Answer from the drawing. Dimensions are ordinates in mm from the lowest x, y and z of the part. A direction names the side the tool comes from. Coordinates: 2 decimals unless noted, no trailing zeros. Order: outer loops, then holes, each group sorted by start corner. A loop starts at its lowest first (then second) coordinate and runs counter-clockwise, first axis right, second up. Notation, with made-up numbers: (80, 75) - (131, 75) arc R33 cw to (131, 103) - close; hole circle Ø9 at (-11.75, -1.5). An arc over 180 degrees is marked (long way). Use CSV: the item, a comma, the result in double quotes. Start each with the question number.
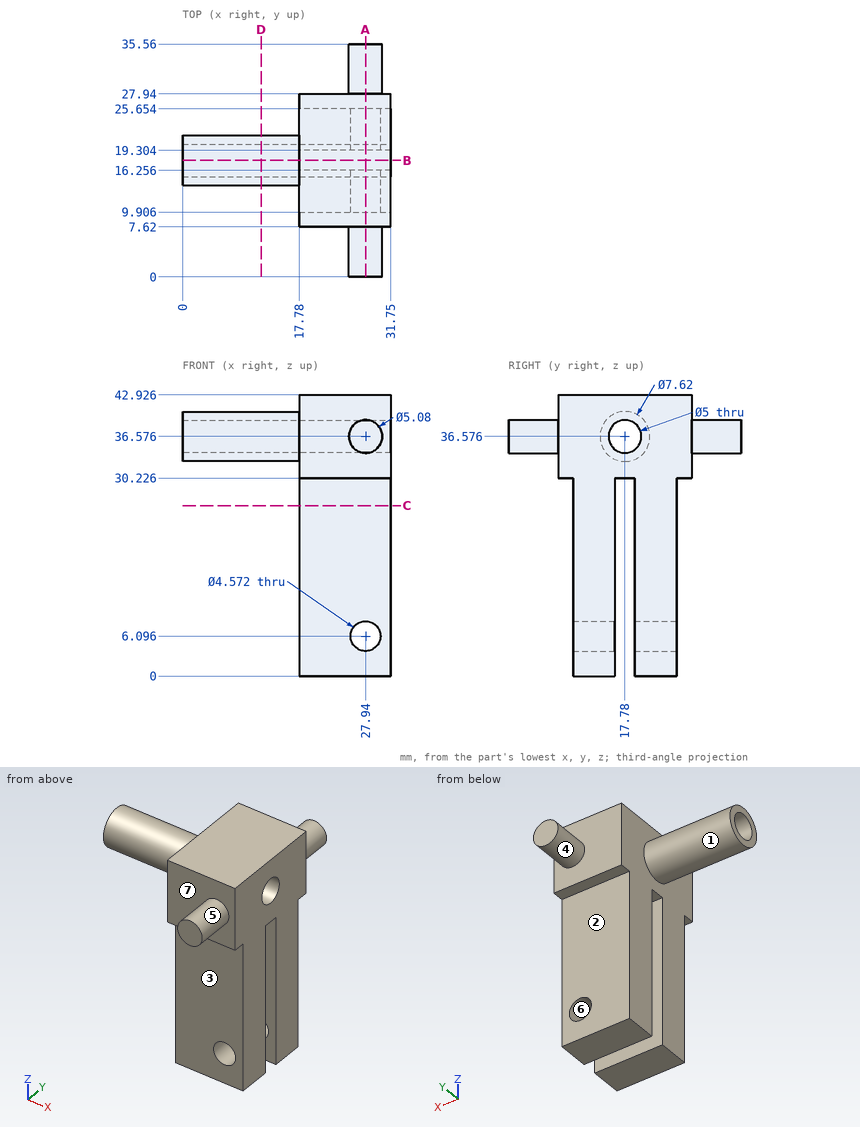
1) Straight lines are drawn through the part: line 1 (Y direction, x = 26, z = 16); line 2 (Z direction, x = 28, y = 13); line 3 (X direction, y = 10, z = 13). For each, find the intervals that lie inside material, in ascending order. Write a range as [from, to].
2) The part is cut by section A-A on x = 27.94. State how many separate pieces and enclosed holes the cut face has, plus the area to 3 significant figures.
3) The part is cut by section C-C on z = 26. Determine the outline of the cut face in (x, y).
4) For the marked faces 1, 2, 3 and 4, determine the directions among +Z, -Z, +X, -X, +Y, -Y from which every point of the face is accessible in a straight line to the end or side of a thin tool.
5) The part is cut by section D-D on x = 12. Determine the outline of the cut face in (y, z), plus the area to 3 significant figures.
6) For a pull along Z with two mould halves and no side action, classify the marked faces 5, 6 and 7 as +Z half, -Z half, draft (parallel to the pull), parting line (faces both ways), or undercut.
7) Flat-ended cylindrical pins translate along their axes: P1, Ø5, axis at x = 8, y = 26.5, coming from the +Z side; P2, Ø11, axis at x = 23.5, z = 15.5, coming from the +Y side; P3, Ø4, axis at y = 24.5, z = 20.5, coming from the -X side; P4, Ø4, axis at x = 24, z = 20.5, coming from the -Y side. Find the tip coordinate at first contact, or state that the pin passes through.
8) The part is cut by section B-B on y = 17.78. Determine the outline of the cut face in (x, z), plus the area to 3 significant figures.
Answer key:
1,line 1,"[9.91, 16.26], [19.3, 25.65]"
1,line 2,"[0, 3.81], [8.38, 42.93]"
1,line 3,"[17.78, 31.75]"
2,separate pieces,"3"
2,enclosed holes,"1"
2,area,"642 mm^2"
3,outline,"(17.78, 9.91) - (31.75, 9.91) - (31.75, 16.26) - (17.78, 16.26) - close; (17.78, 19.3) - (31.75, 19.3) - (31.75, 25.65) - (17.78, 25.65) - close"
4,face 1,"-X"
4,face 2,"-Z, +X, -X, +Y"
4,face 3,"-Z, +X, -X, -Y"
4,face 4,"+Y"
5,outline,"circle Ø7.62 at (17.78, 36.58); hole circle Ø5 at (17.78, 36.58)"
5,area,"26.0 mm^2"
6,face 5,"parting line"
6,face 6,"undercut"
6,face 7,"draft"
7,P1,"through"
7,P2,"y = 25.65"
7,P3,"x = 17.78"
7,P4,"y = 9.91"
8,outline,"(0, 32.77) - (17.78, 32.77) - (17.78, 30.23) - (31.75, 30.23) - (31.75, 34.08) - (0, 34.08) - close; (0, 39.08) - (31.75, 39.08) - (31.75, 42.93) - (17.78, 42.93) - (17.78, 40.39) - (0, 40.39) - close"
8,area,"154 mm^2"
